Design review of the part shown in the three views and the two pictorial views. Dimensions are in mm from the part's minimum x, y and z. A direction names the side the tool comes from. Coordinates: 2 decimals unless noted, no trailing zeros. Loops run counter-clockwise (first coordinate to the right, second up) from the corner with the lowest first, then second, coordinate; pieces in that order, holes last. Notation, with made-up numbers: (70, 48) -> (95, 48) arc R37 cw to (95, 87) -> close; hole circle Ø10 at (54, 25). An arc over 180 degrees is marked (long way). Use CSV: the item, a comma, the result in double quotes.
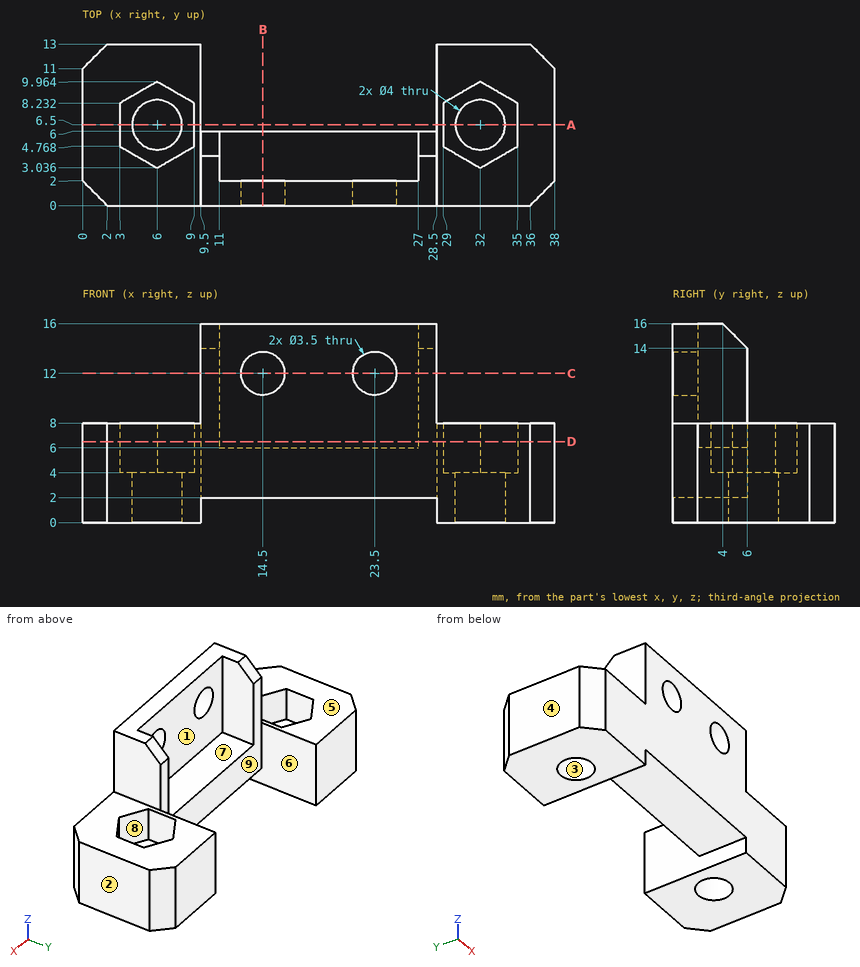
Item 1: Add section C-C (z = 12). Give the boundary of the cut face in (x, y).
Checked values:
outline,"(9.5, 0) -> (12.75, 0) -> (12.75, 2) -> (11, 2) -> (11, 6) -> (9.5, 6) -> close; (16.25, 0) -> (21.75, 0) -> (21.75, 2) -> (16.25, 2) -> close; (25.25, 0) -> (28.5, 0) -> (28.5, 6) -> (27, 6) -> (27, 2) -> (25.25, 2) -> close"
Item 2: Add section D-D (z = 6.5). Give the boundary of the cut face in (x, y).
Checked values:
outline,"(0, 2) -> (2, 0) -> (36, 0) -> (38, 2) -> (38, 11) -> (36, 13) -> (28.5, 13) -> (28.5, 6) -> (27, 6) -> (27, 2) -> (11, 2) -> (11, 6) -> (9.5, 6) -> (9.5, 13) -> (2, 13) -> (0, 11) -> close; hole (3, 4.77) -> (6, 3.04) -> (9, 4.77) -> (9, 8.23) -> (6, 9.96) -> (3, 8.23) -> close; hole (29, 4.77) -> (32, 3.04) -> (35, 4.77) -> (35, 8.23) -> (32, 9.96) -> (29, 8.23) -> close"
Item 3: Clearance check with flat-ended pins moving along their axes: pin 1 (4 mm diameter, centred on x = 32, y = 1.5, fed in from -Z); pin 2 (6.5 mm diameter, centred on x = 20.5, y = 2.5, fed in from -Z); pin 3 (8 mm diameter, centred on x = 22.5, z = 10.5, fed in from +Y); pin 4 (2 mm diameter, centred on y = 3, z = 11, fed in from -X). State where each tip first meets the part, or that it passes through.
Checked values:
pin 1,"z = 0"
pin 2,"z = 2"
pin 3,"y = 2"
pin 4,"x = 9.5"
Item 4: Add section A-A (y = 6.5). Give the boundary of the cut face in (x, z).
Checked values:
outline,"(0, 0) -> (4, 0) -> (4, 4) -> (3, 4) -> (3, 8) -> (0, 8) -> close; (8, 0) -> (9.5, 0) -> (9.5, 8) -> (9, 8) -> (9, 4) -> (8, 4) -> close; (28.5, 0) -> (30, 0) -> (30, 4) -> (29, 4) -> (29, 8) -> (28.5, 8) -> close; (34, 0) -> (38, 0) -> (38, 8) -> (35, 8) -> (35, 4) -> (34, 4) -> close"
Item 5: Machinability: for the marked faces 5, 6, 7, 8 and 9, which of the approach directions +Z, -Z, +X, -X, +Y, -Y give a long, thin tool a straight path to every point of the face, cutting with its end or side? Answer none if there is none.
Checked values:
face 5,"+Z, -X, +Y, -Y"
face 6,"-Z, +Y"
face 7,"+Z, +Y"
face 8,"+Z"
face 9,"+Z, -Z, +Y"
Item 6: Draft analysis for pull direction X (two halves, no side actions). For the marked faces 1, 2, 3 and 4, state which applies: pulls with the +X half, pulls with the -X half, needs draft (parallel to the pull), parting line crosses it, or undercut.
Checked values:
face 1,"undercut"
face 2,"pulls with the +X half"
face 3,"undercut"
face 4,"pulls with the -X half"
Item 7: Add section B-B (x = 14.5). Give the boundary of the cut face in (y, z).
Checked values:
outline,"(0, 2) -> (6, 2) -> (6, 6) -> (2, 6) -> (2, 10.25) -> (0, 10.25) -> close; (0, 13.75) -> (2, 13.75) -> (2, 16) -> (0, 16) -> close"
Item 8: To check wall thickness, follow line 1 along X through (y, z) = (1.45, 12); line 2 along X through (y, z) = (5.25, 4.5); line 3 along X through (y, z) = (6.25, 3). State the ranges of each line that lie inside material, in increasing order.
Checked values:
line 1,"9.5 to 12.75, 16.25 to 21.75, 25.25 to 28.5"
line 2,"0 to 3, 9 to 29, 35 to 38"
line 3,"0 to 4.02, 7.98 to 9.5, 28.5 to 30.02, 33.98 to 38"
